from build123d import *

# Parameters (mm, degrees)
SKETCH1_W           = 228.6
SKETCH1_H           = 107.95
SKETCH1_W_2         = 76.2
SKETCH1_H_2         = 6.35
SKETCH1_W_3         = 6.35
SKETCH1_H_3         = 76.2
BOSS_EXTRUDE1_DEPTH = 6.35


with BuildPart() as part:
    # Sketch1 → Boss-Extrude1 (new body)
    with BuildSketch(Plane.XY):
        with Locations((64.733678216, -34.923106362)):
            Rectangle(SKETCH1_W, SKETCH1_H)
        with Locations((64.733678216, 22.226893638)):
            Rectangle(SKETCH1_W_2, SKETCH1_H_2)
        Polygon((185.383678216, -69.848106362), (185.383678216, 2.969008236), (185.383678216, 6.351893638), (179.033678216, 6.351893638), (179.033678216, -69.848106362), align=None)
        with Locations((-52.741321784, -31.748106362)):
            Rectangle(SKETCH1_W_3, SKETCH1_H_3)
    extrude(amount=BOSS_EXTRUDE1_DEPTH)


solid = part.part
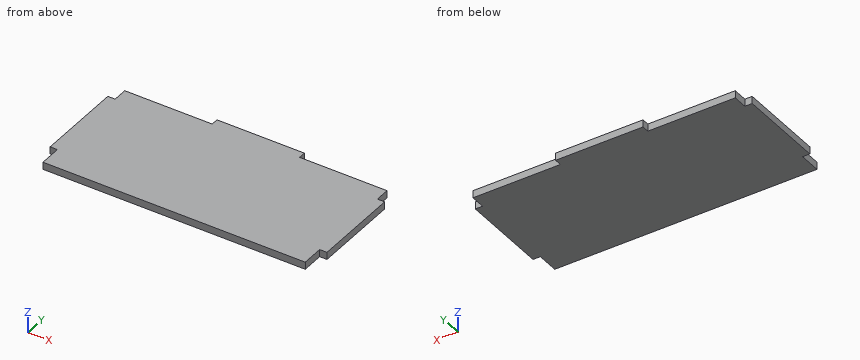
Verification items for the finished model (mm, model axes). Give positions to 0.01 mm unless a question says otherwise; leave off trailing zeros. Order: outer loops, then holes, each group sorted by start corner. A loop starts at its lowest first (then second) coordinate and runs counter-clockwise, first axis right, second up. Notation, with made-up numbers: M -18,30 L 26,30 A29 cw 26,55 Z; hole C 39.5,8 d4. An arc over 180 degrees is marked long. Answer as a JSON object with one key per item and string values. Group by question number.
1) Scan lines: line 1 along Y through (x, z) = (-33.5, 4.5); line 2 along X through (y, z) = (16, 4). Record each from-to range of solid material in increasing order. Write a range as [from, to].
2) Depth check by flat-ended pin: pin 1 Ø1.9 at (y, z) = (23.5, 4.5) entering from +X; pin 2 Ø1 at (x, z) = (126, 1) entering from +Y; pin 3 Ø3 at (y, z) = (9.5, 2.5) entering from +X. Enter the tip coordinate at first touch or a pass-through.
3) Cross-section at A-A (z = 1.25). Enter the section's corners in (x, y), then the cut area to 3 significant figures.
4) Cross-section at B-B (x = 106). Enter the section's corners in (y, z), then the cut area to 3 significant figures.
5) Cross-section at C-C (y = -82). Enter the section's corners in (x, z).
Result sheet:
{
 "1": {"line 1": "y = [-88.9, 19.05]", "line 2": "x = [-49.57, 179.03]"},
 "2": {"pin 1": "stops at x = 102.83", "pin 2": "stops at y = 19.05", "pin 3": "stops at x = 179.03"},
 "3": {"outline": "M -55.92,-69.85 L -49.57,-69.85 L -49.57,-88.9 L 179.03,-88.9 L 179.03,-69.85 L 185.38,-69.85 L 185.38,6.35 L 179.03,6.35 L 179.03,19.05 L 102.83,19.05 L 102.83,25.4 L 26.63,25.4 L 26.63,19.05 L -49.57,19.05 L -49.57,6.35 L -55.92,6.35 Z", "area": "26,100 mm2"},
 "4": {"outline": "M -88.9,0 L 19.05,0 L 19.05,6.35 L -88.9,6.35 Z", "area": "685 mm2"},
 "5": {"outline": "M -49.57,0 L 179.03,0 L 179.03,6.35 L -49.57,6.35 Z"}
}
